```python
from build123d import *

# Parameters (mm, degrees)
SKETCH_W      = 44
SKETCH_H      = 53
SKETCH_R      = 1.65
SKETCH_R_2    = 0.5
PAD_DEPTH     = 2
SKETCH001_R   = 0.5
SKETCH001_W   = 15
SKETCH001_H   = 25
SKETCH001_W_2 = 22.5
SKETCH001_H_2 = 53
PAD001_DEPTH  = 2


with BuildPart() as part:
    # Sketch → Pad (new body)
    with BuildSketch(Plane.XY):
        with Locations((16, 26.5)):
            Rectangle(SKETCH_W, SKETCH_H)
        with Locations((13.5, 43)):
            Circle(SKETCH_R, mode=Mode.SUBTRACT)
        with Locations((13.5, 33)):
            Circle(SKETCH_R, mode=Mode.SUBTRACT)
        with Locations((1, 50.5)):
            Circle(SKETCH_R_2, mode=Mode.SUBTRACT)
        with Locations((3.5, 50.5)):
            Circle(SKETCH_R_2, mode=Mode.SUBTRACT)
        with Locations((6, 50.5)):
            Circle(SKETCH_R_2, mode=Mode.SUBTRACT)
        with Locations((8.5, 50.5)):
            Circle(SKETCH_R_2, mode=Mode.SUBTRACT)
        with Locations((11, 50.5)):
            Circle(SKETCH_R_2, mode=Mode.SUBTRACT)
        with Locations((13.5, 50.5)):
            Circle(SKETCH_R_2, mode=Mode.SUBTRACT)
        with Locations((-4, 50.5)):
            Circle(SKETCH_R_2, mode=Mode.SUBTRACT)
        with Locations((-1.5, 50.5)):
            Circle(SKETCH_R_2, mode=Mode.SUBTRACT)
        with Locations((8.75, 4.5)):
            Circle(SKETCH_R_2, mode=Mode.SUBTRACT)
        with Locations((11.25, 4.5)):
            Circle(SKETCH_R_2, mode=Mode.SUBTRACT)
        with Locations((3.75, 4.5)):
            Circle(SKETCH_R_2, mode=Mode.SUBTRACT)
        with Locations((6.25, 4.5)):
            Circle(SKETCH_R_2, mode=Mode.SUBTRACT)
        with Locations((8.75, 2)):
            Circle(SKETCH_R_2, mode=Mode.SUBTRACT)
        with Locations((11.25, 2)):
            Circle(SKETCH_R_2, mode=Mode.SUBTRACT)
        with Locations((3.75, 2)):
            Circle(SKETCH_R_2, mode=Mode.SUBTRACT)
        with Locations((6.25, 2)):
            Circle(SKETCH_R_2, mode=Mode.SUBTRACT)
    extrude(amount=PAD_DEPTH)

    # Sketch001 → Pad001 (join)
    with BuildSketch(Plane.XY.offset(1.5)):
        with Locations((1, 50.5)):
            Circle(SKETCH001_R)
        with Locations((3.5, 50.5)):
            Circle(SKETCH001_R)
        with Locations((6, 50.5)):
            Circle(SKETCH001_R)
        with Locations((8.5, 50.5)):
            Circle(SKETCH001_R)
        with Locations((11, 50.5)):
            Circle(SKETCH001_R)
        with Locations((13.5, 50.5)):
            Circle(SKETCH001_R)
        with Locations((-4, 50.5)):
            Circle(SKETCH001_R)
        with Locations((-1.5, 50.5)):
            Circle(SKETCH001_R)
        with Locations((7.5, 12.5)):
            Rectangle(SKETCH001_W, SKETCH001_H)
        with Locations((8.75, 4.5)):
            Circle(SKETCH001_R, mode=Mode.SUBTRACT)
        with Locations((11.25, 4.5)):
            Circle(SKETCH001_R, mode=Mode.SUBTRACT)
        with Locations((3.75, 4.5)):
            Circle(SKETCH001_R, mode=Mode.SUBTRACT)
        with Locations((6.25, 4.5)):
            Circle(SKETCH001_R, mode=Mode.SUBTRACT)
        with Locations((8.75, 2)):
            Circle(SKETCH001_R, mode=Mode.SUBTRACT)
        with Locations((11.25, 2)):
            Circle(SKETCH001_R, mode=Mode.SUBTRACT)
        with Locations((3.75, 2)):
            Circle(SKETCH001_R, mode=Mode.SUBTRACT)
        with Locations((6.25, 2)):
            Circle(SKETCH001_R, mode=Mode.SUBTRACT)
        with Locations((26.75, 26.5)):
            Rectangle(SKETCH001_W_2, SKETCH001_H_2)
    extrude(amount=PAD001_DEPTH)


solid = part.part
```
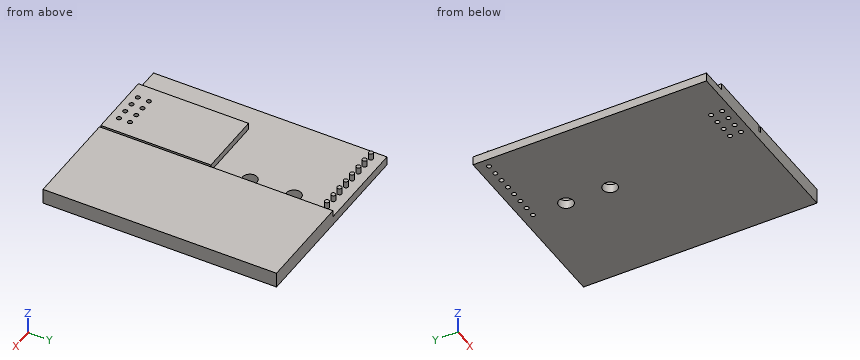
Geometry: final body of the model. Coordinates: model frame, mm. Round coordinates to 2 decimals unless told otherwise and drop trailing zeros. Write each loop counter-clockwise with the first axis right and the second up, starting at its lowest first coordinate (ties: lowest second). Pieces come first, ordered by that corner, then holes.
Item 1: Pin query (flat end, axial travel): P1, Ø0.8, axis at x = 3.5, y = 50.5, coming from the -Z side; P2, Ø3, axis at x = 13.5, y = 43, coming from the +Z side. Return the tip coordinate at first contact, or that it passes through.
Item 2: Material intervals for L1, parallel to X at y = 9, z = 2.75; L2, parallel to Y at x = 7.5, z = 2.2; L3, parallel to X at y = 48, z = 2.05, sorted ascending.
Item 3: Section query A-A (y = 43). Return loops of the section in (x, z), plus the area to 3 significant figures.
Completed:
1. P1: stops at z = 1.5
1. P2: passes through
2. L1: x = 0 to 15, 15.5 to 38
2. L2: y = 0 to 25
2. L3: x = 15.5 to 38
3. outline: (-6, 0) - (11.85, 0) - (11.85, 2) - (-6, 2) - close; (15.15, 0) - (38, 0) - (38, 3.5) - (15.5, 3.5) - (15.5, 2) - (15.15, 2) - close
3. area: 115 mm2
